```python
from build123d import *

# Parameters (mm, degrees)
SKETCH1_R              = 12.7
BOSS_EXTRUDE1_DEPTH    = 292.1
CUT_EXTRUDE2_START     = -12.700000102
CUT_EXTRUDE2_OUTLINE_R = 3.175
CUT_EXTRUDE2_DEPTH     = 25.400000102


# Read off the part's stored shape, not the designer's step: Cut-Extrude2
with BuildPart() as part:
    # Sketch1 → Boss-Extrude1 (new, symmetric)
    with BuildSketch(Plane.XY):
        Circle(SKETCH1_R)
    extrude(amount=BOSS_EXTRUDE1_DEPTH, both=True)

    # Cut-Extrude2 outline → Cut-Extrude2 (cut)
    with BuildSketch(Plane(origin=(0, 0, 0), x_dir=(0, 0, -1), z_dir=(1, 0, 0)).offset(CUT_EXTRUDE2_START)):
        with BuildLine():
            ThreePointArc((-292.1, 3.2e-08), (-288.38025611, 8.980256132), (-279.4, 12.7))
            Line((-279.4, 12.7), (-292.1, 12.7))
            Line((-292.1, 12.7), (-292.1, 3.2e-08))
        make_face()
        with BuildLine():
            Line((292.1, 12.7), (279.4, 12.7))
            ThreePointArc((279.4, 12.7), (288.38025611, 8.980256132), (292.1, 3.2e-08))
            Line((292.1, 3.2e-08), (292.1, 12.7))
        make_face()
        with BuildLine():
            ThreePointArc((-279.4, -12.7), (-288.380256132, -8.98025611), (-292.1, 3.2e-08))
            Line((-292.1, 3.2e-08), (-292.1, -12.7))
            Line((-292.1, -12.7), (-279.4, -12.7))
        make_face()
        with BuildLine():
            Line((292.1, -12.7), (292.1, 3.2e-08))
            ThreePointArc((292.1, 3.2e-08), (288.380256132, -8.98025611), (279.4, -12.7))
            Line((279.4, -12.7), (292.1, -12.7))
        make_face()
        with Locations((-279.4, 0)):
            Circle(CUT_EXTRUDE2_OUTLINE_R)
        with Locations((279.4, 0)):
            Circle(CUT_EXTRUDE2_OUTLINE_R)
    extrude(amount=CUT_EXTRUDE2_DEPTH, mode=Mode.SUBTRACT)


solid = part.part
```
Geometry check sheet. Reference: the model listing, model coordinates, mm. Coordinates: 2 decimals unless noted, no trailing zeros. Order: outer loops, then holes, each group sorted by start corner. A loop starts at its lowest first (then second) coordinate and runs counter-clockwise, first axis right, second up. Notation, with made-up numbers: (5, -25.5) - (56, -25.5) arc R19 ccw to (56, -15.5) - close; hole circle Ø10 at (85, 0.25). An arc over 180 degrees is marked (long way). Answer in a Markdown table with one row per item. Add a question column.
1. Gauge pin test, flat ends, axial feed: pin 1 Ø1.5 at (x, y) = (-4.5, -3) entering from +Z; pin 2 Ø1 at (x, z) = (-2, -104.5) entering from -Y; pin 3 Ø4 at (x, z) = (3, 64.5) entering from +Y; pin 4 Ø12 at (y, z) = (-1, 222.5) entering from +X. Record the tip position at first contact, or that the pin passes through.
2. Section check A-A (x = 5). Enter the section's corners in (y, z) (3 decimals).
3. Section check B-B (z = 50.5). Enter the section's corners in (x, y), plus the area to 3 significant figures.
4. Material ranges on L1, parallel to Y at x = -1.25, z = 279.4 (3 decimals); L2, parallel to Z at x = -11, y = 1.5; L3, parallel to Y at x = 0.25, z = -279.4 (3 decimals), recorded low to high. Write a range as [from, to].
5. Section check C-C (y = -8.75). Enter the section's corners in (x, z).
Data:
| question | item | result |
|---|---|---|
| 1 | pin 1 | stops at z = 291.9 |
| 1 | pin 2 | stops at y = -12.61 |
| 1 | pin 3 | stops at y = 12.66 |
| 1 | pin 4 | stops at x = 12.7 |
| 2 | outline | (-11.674, -284.4) arc R12.7 ccw to (11.674, -284.4) - (11.674, 284.4) arc R12.7 ccw to (-11.674, 284.4) - close; hole circle Ø6.35 at (0, -279.4); hole circle Ø6.35 at (0, 279.4) |
| 3 | outline | circle Ø25.4 at (0, 0) |
| 3 | area | 507 mm² |
| 4 | L1 | y = [-12.638, -3.175], [3.175, 12.638] |
| 4 | L2 | z = [-292.01, -282.2], [-276.6, 276.6], [282.2, 292.01] |
| 4 | L3 | y = [-12.698, -3.175], [3.175, 12.698] |
| 5 | outline | (-9.2, -288.6) - (9.2, -288.6) - (9.2, 288.6) - (-9.2, 288.6) - close |
